Design review of the part shown in the three views and the two pictorial views. Dimensions are in mm from the part's minimum x, y and z. A direction names the side the tool comes from. Round coordinates to 2 decimals unless told otherwise and drop trailing zeros. Loops run counter-clockwise (first coordinate to the right, second up) from the corner with the lowest first, then second, coordinate; pieces in that order, holes last. Notation, with made-up numbers: (-39.75, -22.75) - (-34.75, -22.75) arc R12 cw to (-34.75, -4.75) - close; hole circle Ø5 at (20.5, -6.5). An arc over 180 degrees is marked (long way). Return JSON: item names as keys, results as strings. Group by question number.
(1) We need section D-D, the plane x = 93. Write out the cut boundary in (y, z) (3 decimals).
(2) Wall thickness on L1, parallel to X at y = 1.25, z = 27.94; L2, parallel to X at y = 6.25, z = 68; L3, parallel to Z at x = 14, y = 13.25 (3 decimals): over which ranges is each line inside the solid? List them lowest first. Write a range as [from, to].
(3) The part is to be moulded in two halves that separate along X. For the marked faces 3, 4 and 5, say which applies: pulls with the +X half, pulls with the -X half, needs draft (parallel to the pull), parting line crosses it, or undercut.
(4) Clearance check with flat-ended pins moving along their axes: pin 1 (1 mm diameter, centred on x = 77.5, y = 12.5, fed in from -Z); pin 2 (2.5 mm diameter, centred on x = 5.08, z = 6.731, fed in from +Y) (3 decimals). State where each tip first meets the part, or that it passes through.
(5) We need section C-C, the plane z = 20. Write out the cut boundary in (x, y) (3 decimals), and give its area (3 significant figures).
(6) For the marked faces 1 and 2, list the 3-axis set-ups (+Z, -Z, +X, -X, +Y, -Y) from which the entire face can be reached by the end or side of a thin tool; tool diameter is ignored.
(7) We need section B-B, the plane y = 9. Write out the cut boundary in (x, z) (3 decimals), and give its area (3 significant figures).
(8) We need section A-A, the plane z = 48.26. Write out the cut boundary in (x, y) (1 decimal).
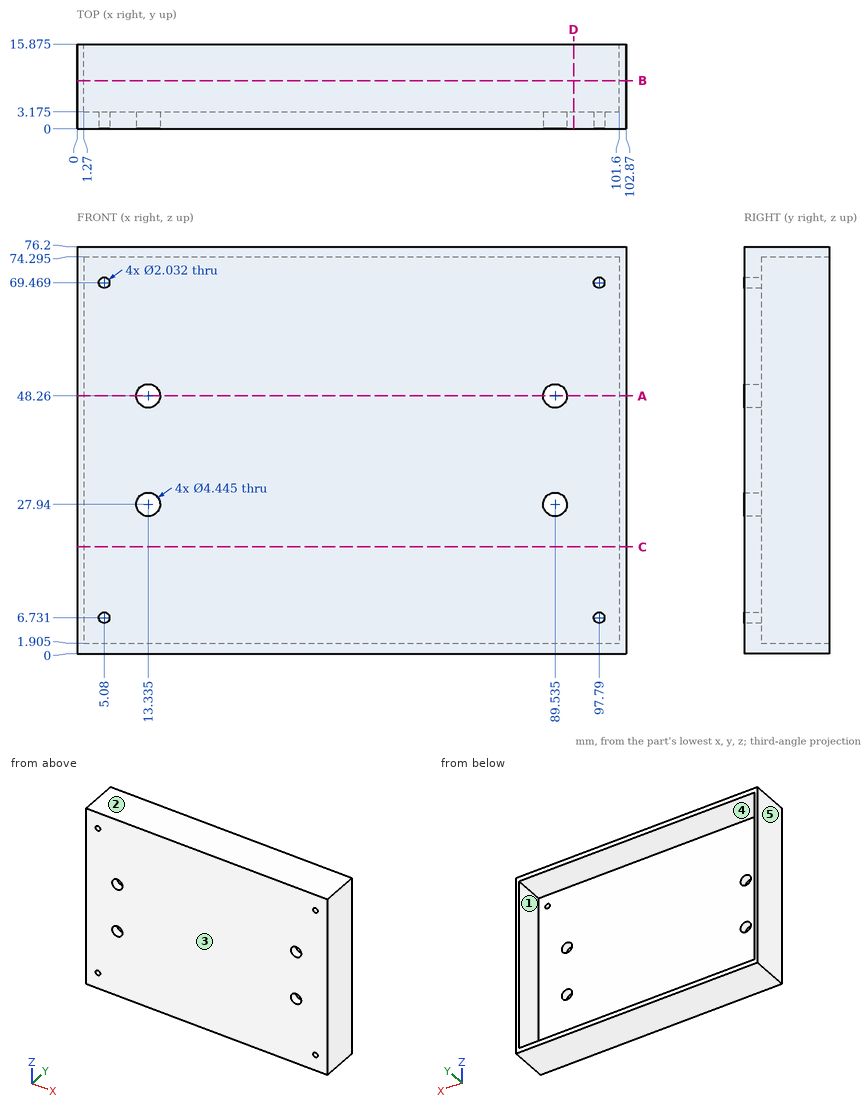
Solutions:
{
 "1": {"outline": "(0, 0) - (15.875, 0) - (15.875, 1.905) - (3.175, 1.905) - (3.175, 74.295) - (15.875, 74.295) - (15.875, 76.2) - (0, 76.2) - close"},
 "2": {"L1": "[0, 11.11], [15.56, 87.31], [91.76, 102.87]", "L2": "[0, 1.27], [101.6, 102.87]", "L3": "[0, 1.905], [74.295, 76.2]"},
 "3": {"face 3": "needs draft", "face 4": "undercut", "face 5": "pulls with the -X half"},
 "4": {"pin 1": "z = 0", "pin 2": "y = 3.175"},
 "5": {"outline": "(0, 0) - (102.87, 0) - (102.87, 15.875) - (101.6, 15.875) - (101.6, 3.175) - (1.27, 3.175) - (1.27, 15.875) - (0, 15.875) - close", "area": "359 mm^2"},
 "6": {"face 1": "+Y", "face 2": "+Z, +X, -X, +Y, -Y"},
 "7": {"outline": "(0, 0) - (102.87, 0) - (102.87, 76.2) - (0, 76.2) - close; hole (1.27, 1.905) - (101.6, 1.905) - (101.6, 74.295) - (1.27, 74.295) - close", "area": "576 mm^2"},
 "8": {"outline": "(0, 0) - (11.1, 0) - (11.1, 3.2) - (1.3, 3.2) - (1.3, 15.9) - (0, 15.9) - close; (15.6, 0) - (87.3, 0) - (87.3, 3.2) - (15.6, 3.2) - close; (91.8, 0) - (102.9, 0) - (102.9, 15.9) - (101.6, 15.9) - (101.6, 3.2) - (91.8, 3.2) - close"}
}
